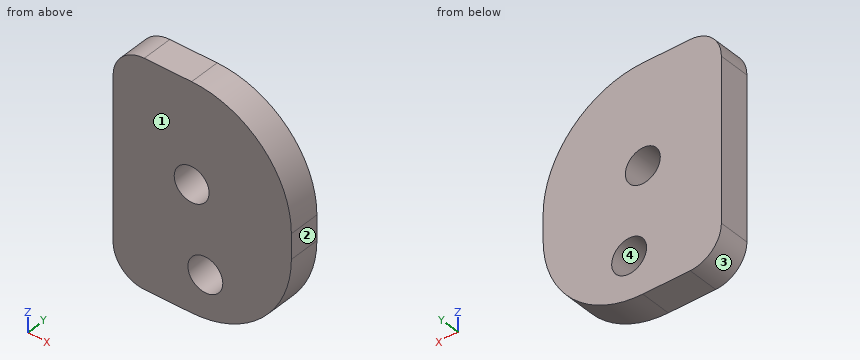
from build123d import *

# Parameters (mm, degrees)
SKETCH1_W           = 50.8
SKETCH1_H           = 22.86
BOSS_EXTRUDE1_DEPTH = 3.175
FILLET1_R           = 10.16
SKETCH3_R           = 1.778
CUT_EXTRUDE1_DEPTH  = 29.033649869
FILLET3_R           = 10.16
SKETCH4_W           = 32.639
SKETCH4_H           = 22.86
CUT_EXTRUDE2_DEPTH  = 29.033649869
FILLET9_R           = 3.175


with BuildPart() as part:
    # Sketch1 → Boss-Extrude1 (new body)
    with BuildSketch(Plane(origin=(0, 0, 0), x_dir=(1, 0, 0), z_dir=(0, 1, 0))):
        Rectangle(SKETCH1_W, SKETCH1_H)
    extrude(amount=BOSS_EXTRUDE1_DEPTH)

    # Fillet1
    fillet1_edges = [part.edges().sort_by_distance(p)[0] for p in [
        (25.4, 1.5875, 11.43),
        (-25.4, 1.5875, 11.43),
    ]]
    fillet(fillet1_edges, radius=FILLET1_R)

    # Sketch3 → Cut-Extrude1 (cut, through all)
    with BuildSketch(Plane(origin=(0, 3.175, 0), x_dir=(1, 0, 0), z_dir=(0, 1, 0))):
        with Locations(Location((15.24, -1.27, 0), (0, 0, 270))):
            Circle(SKETCH3_R)
        with Locations(Location((16.637, 6.994763457, 0), (0, 0, 270))):
            Circle(SKETCH3_R)
        with Locations(Location((-3.81, -1.27, 0), (0, 0, 270))):
            Circle(SKETCH3_R)
    extrude(amount=-CUT_EXTRUDE1_DEPTH, mode=Mode.SUBTRACT)

    # Fillet3
    fillet3_edges = [part.edges().sort_by_distance(p)[0] for p in [
        (-25.4, 1.5875, -11.43),
        (25.4, 1.5875, -11.43),
    ]]
    fillet(fillet3_edges, radius=FILLET3_R)

    # Sketch4 → Cut-Extrude2 (cut, through all)
    with BuildSketch(Plane(origin=(0, 3.175, 0), x_dir=(1, 0, 0), z_dir=(0, 1, 0))):
        with Locations((-9.0805, 0)):
            Rectangle(SKETCH4_W, SKETCH4_H)
    extrude(amount=-CUT_EXTRUDE2_DEPTH, mode=Mode.SUBTRACT)

    # Fillet9
    fillet9_edges = [part.edges().sort_by_distance(p)[0] for p in [
        (7.239, 1.5875, -11.43),
        (7.239, 1.5875, 11.43),
    ]]
    fillet(fillet9_edges, radius=FILLET9_R)


solid = part.part
For this review, take the finished solid that the model builds, in its own axes (mm). Face numbers are marked on the shaded views. Round coordinates to 2 decimals unless told otherwise and drop trailing zeros. Loops run counter-clockwise (first coordinate to the right, second up) from the corner with the lowest first, then second, coordinate; pieces in that order, holes last. Notation, with made-up numbers: (-26.5, 53) - (24.5, 53) arc R16 ccw to (24.5, 80) - close; hole circle Ø2 at (77.25, -20.75). An arc over 180 degrees is marked (long way). Put each result on its own line as item: value. Start each with the question number.
1. Consider section D-D on z = 8.75. State the section outline as (x, y) points (3 decimals), plus the area to 3 significant figures.
2. Mouldability with a two-part tool opening along X and no side actions: class the marked faces 1, 2, 3 and 4 as +X half, -X half, draft (parallel to the pull), parting line (faces both ways), or undercut.
3. For probe 1 along Z at (x, y) = (15.25, 2); probe 2 along X at (y, z) = (0.5, -5.75); probe 3 along X at (y, z) = (1.2, 2.5), list the stretches that pass through material, from the lowest coordinate up. Write a range as [from, to].
4. Consider section C-C on x = 13.75. State the section outline as (y, z) points (3 decimals), plus the area to 3 significant figures.
5. Consider section B-B on y = 1.35. State the section outline as (x, z) points (3 decimals), plus the area to 3 significant figures.
6. Consider section A-A on x = 15.75. State the section outline as (y, z) points (3 decimals).
Result sheet:
1. outline: (7.278, 0) - (22.116, 0) - (22.116, 3.175) - (7.278, 3.175) - close
1. area: 47.1 mm^2
2. face 1: draft
2. face 2: +X half
2. face 3: -X half
2. face 4: undercut
3. probe 1: [-11.43, -8.11], [-5.88, -0.51], [3.05, 11.43]
3. probe 2: [7.24, 15.37], [17.91, 24.36]
3. probe 3: [7.24, 13.96], [16.52, 25.33]
4. outline: (0, -11.43) - (3.175, -11.43) - (3.175, 0.3) - (0, 0.3) - close; (0, 2.24) - (3.175, 2.24) - (3.175, 11.43) - (0, 11.43) - close
4. area: 66.4 mm^2
5. outline: (7.239, -8.255) arc R3.175 ccw to (10.414, -11.43) - (15.24, -11.43) arc R10.16 ccw to (25.4, -1.27) - (25.4, 1.27) arc R10.16 ccw to (15.24, 11.43) - (10.414, 11.43) arc R3.175 ccw to (7.239, 8.255) - close; hole circle Ø3.556 at (15.24, 1.27); hole circle Ø3.556 at (16.637, -6.995)
5. area: 347 mm^2
6. outline: (0, -11.417) - (3.175, -11.417) - (3.175, -8.536) - (0, -8.536) - close; (0, -5.454) - (3.175, -5.454) - (3.175, -0.433) - (0, -0.433) - close; (0, 2.973) - (3.175, 2.973) - (3.175, 11.417) - (0, 11.417) - close
